```python
from build123d import *

# Parameters (mm, degrees)
F0_W     = 64.15522
F0_H     = 76.186978
F1_DEPTH = 72
F2_T     = -13
F3_R     = 12.673709
F4_DEPTH = 108.5


with BuildPart() as f1:
    # F0 (on Top) → F1 (new body)
    with BuildSketch(Plane.XY):
        Rectangle(F0_W, F0_H)
    extrude(amount=F1_DEPTH)

    # F2
    f2_openings = [f1.faces().sort_by_distance(p)[0] for p in [
        (0, 0, 72),
    ]]
    offset(amount=F2_T, openings=f2_openings)

    # F3 (on face) → F4 (cut)
    with BuildSketch(Plane.XZ.offset(38.093489)):
        with Locations((0, 36)):
            Circle(F3_R)
    extrude(amount=-F4_DEPTH, mode=Mode.SUBTRACT)


solid = f1.part
```
The model under review builds one solid part; all positions refer to its coordinate system, in mm. A direction names the side the tool comes from. Round coordinates to 2 decimals unless told otherwise and drop trailing zeros. Order: outer loops, then holes, each group sorted by start corner. A loop starts at its lowest first (then second) coordinate and runs counter-clockwise, first axis right, second up. Notation, with made-up numbers: (7, 24) -> (25, 24) arc R28 ccw to (25, 55) -> close; hole circle Ø11 at (10, 66.25). An arc over 180 degrees is marked (long way). One line per item, written item: value. Start each with the question number.
Q1. Take a section at D-D (z = 62). Write out the cut boundary in (x, y).
Q2. Take a section at A-A (x = 0). Write out the cut boundary in (y, z), and give its area (3 significant figures).
Q3. Machinability: for faces 4 (the face through (0, 1, 0)), 5 (the face through (19.078, 0, 42)), which of the approach directions +Z, -Z, +X, -X, +Y, -Y give a long, thin tool a straight path to every point of the face, cutting with its end or side? Answer none if there is none.
Q4. Take a section at B-B (z = 36). Write out the cut boundary in (x, y), and give its area (3 significant figures).
Q5. Wall thickness on line 1 (Y direction, x = 14, z = 43); line 2 (X direction, y = 16, z = 51); line 3 (Z direction, x = 0, y = -35.25): over which ranges is each line inside the solid? List them lowest first.
Q6. Take a section at C-C (y = 33.5). Write out the cut boundary in (x, z).
Q7. Mouldability with a two-part tool opening along Y and no side actions: class faces 1 (the face through (0, 0, 13)), 2 (the face through (32.078, -1, 35)), 3 (the face through (-15, -38.093, 35)) as released by +Y, released by -Y, zero draft, split by the parting line, or undercut.
Reported:
1. outline: (-32.08, -38.09) -> (32.08, -38.09) -> (32.08, 38.09) -> (-32.08, 38.09) -> close; hole (-19.08, -25.09) -> (19.08, -25.09) -> (19.08, 25.09) -> (-19.08, 25.09) -> close
2. outline: (-38.09, 0) -> (38.09, 0) -> (38.09, 23.33) -> (25.09, 23.33) -> (25.09, 13) -> (-25.09, 13) -> (-25.09, 23.33) -> (-38.09, 23.33) -> close; (-38.09, 48.67) -> (-25.09, 48.67) -> (-25.09, 72) -> (-38.09, 72) -> close; (25.09, 48.67) -> (38.09, 48.67) -> (38.09, 72) -> (25.09, 72) -> close
2. area: 1,870 mm2
3. face 4: -Z, +X, -X, +Y, -Y
3. face 5: +Z
4. outline: (-32.08, -38.09) -> (-12.67, -38.09) -> (-12.67, -25.09) -> (-19.08, -25.09) -> (-19.08, 25.09) -> (-12.67, 25.09) -> (-12.67, 38.09) -> (-32.08, 38.09) -> close; (12.67, -38.09) -> (32.08, -38.09) -> (32.08, 38.09) -> (12.67, 38.09) -> (12.67, 25.09) -> (19.08, 25.09) -> (19.08, -25.09) -> (12.67, -25.09) -> close
4. area: 2,310 mm2
5. line 1: y = -38.09 to -25.09, 25.09 to 38.09
5. line 2: x = -32.08 to -19.08, 19.08 to 32.08
5. line 3: z = 0 to 23.33, 48.67 to 72
6. outline: (-32.08, 0) -> (32.08, 0) -> (32.08, 72) -> (-32.08, 72) -> close; hole circle Ø25.35 at (0, 36)
7. face 1: undercut
7. face 2: zero draft
7. face 3: released by -Y
